```python
from build123d import *

# Parameters (mm, degrees)
BOSS_EXTRUDE1_DEPTH = 50
CUT_EXTRUDE1_REACH  = 9
SKETCH3_R           = 2.5


with BuildPart() as part:
    # Sketch2 → Boss-Extrude1 (new body)
    with BuildSketch(Plane.XY):
        Polygon((-15.713485752, 63.637116303), (-18.483485752, 60.867117128), (-15.713485752, 58.097116303), (-15.713485752, 51.097116303), (-22.713485752, 51.097116303), (-22.713485752, 65.637116303), (-15.713485752, 65.637116303), align=None)
    extrude(amount=BOSS_EXTRUDE1_DEPTH)

    # Sketch3 → Cut-Extrude1 (cut, up to next)
    with BuildSketch(Plane.ZY.offset(22.713485752), mode=Mode.PRIVATE) as cut_extrude1_sk1:
        with Locations((17, 55.097116303)):
            Circle(SKETCH3_R)
    cut_extrude1_tool1 = extrude(cut_extrude1_sk1.sketch, amount=-CUT_EXTRUDE1_REACH, mode=Mode.PRIVATE) & part.part
    add(cut_extrude1_tool1.solids().sort_by_distance((-22.713486, 55.097116, 17))[0], mode=Mode.SUBTRACT)
    # Sketch3 → Cut-Extrude1 (cut, up to next)
    with BuildSketch(Plane.ZY.offset(22.713485752), mode=Mode.PRIVATE) as cut_extrude1_sk2:
        with Locations((33, 55.097116303)):
            Circle(SKETCH3_R)
    cut_extrude1_tool2 = extrude(cut_extrude1_sk2.sketch, amount=-CUT_EXTRUDE1_REACH, mode=Mode.PRIVATE) & part.part
    add(cut_extrude1_tool2.solids().sort_by_distance((-22.713486, 55.097116, 33))[0], mode=Mode.SUBTRACT)


solid = part.part
```
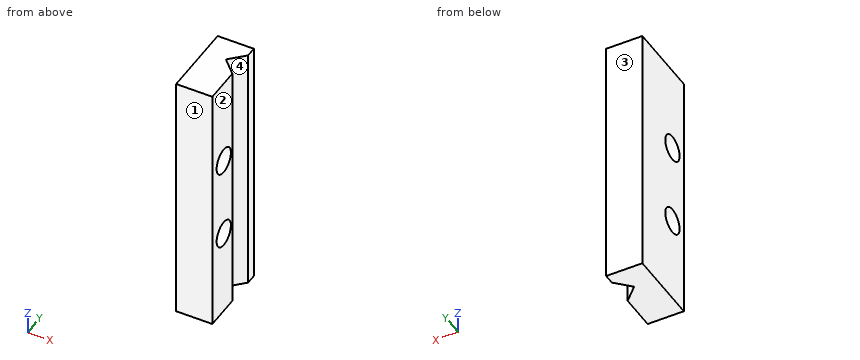
Read the model definition and answer for the solid it produces. Units are mm, in the model's axes. Face numbers are marked on the shaded views. Coordinates: 2 decimals unless noted, no trailing zeros. Loops run counter-clockwise (first coordinate to the right, second up) from the corner with the lowest first, then second, coordinate; pieces in that order, holes last.
(1) Consider line 1 along Y through (x, z) = (-20.5, 17); line 2 along Z through (x, y) = (-18.75, 53.25); line 3 along Z through (x, y) = (-17.25, 54.25). Determine where each line is inside the solid, lowest interval first.
Solution:
line 1: y = 51.1 to 52.6, 57.6 to 65.64
line 2: z = 0 to 15.32, 18.68 to 31.32, 34.68 to 50
line 3: z = 0 to 14.65, 19.35 to 30.65, 35.35 to 50
(2) The mould has two halves that part along Y. Classify the marked faces 1, 2, 3 and 4: released by +Y, released by -Y, zero draft, split by the parting line, or undercut.
Solution:
face 1: released by -Y
face 2: zero draft
face 3: released by +Y
face 4: undercut
(3) The part is cut by section C-C (z = 12). Determine the outline of the cut face in (x, y), and give its area (3 significant figures).
Solution:
outline: (-22.71, 51.1) - (-15.71, 51.1) - (-15.71, 58.1) - (-18.48, 60.87) - (-15.71, 63.64) - (-15.71, 65.64) - (-22.71, 65.64) - close
area: 94.1 mm2
(4) The part is cut by section D-D (y = 62.25). Determine the outline of the cut face in (x, z).
Solution:
outline: (-22.71, 0) - (-17.1, 0) - (-17.1, 50) - (-22.71, 50) - close
(5) The part is cut by section B-B (x = -19.75). Determine the outline of the cut face in (y, z).
Solution:
outline: (51.1, 0) - (65.64, 0) - (65.64, 50) - (51.1, 50) - close; hole circle Ø5 at (55.1, 17); hole circle Ø5 at (55.1, 33)
(6) The part is cut by section A-A (z = 33). Determine the outline of the cut face in (x, y).
Solution:
outline: (-22.71, 51.1) - (-15.71, 51.1) - (-15.71, 52.6) - (-22.71, 52.6) - close; (-22.71, 57.6) - (-15.71, 57.6) - (-15.71, 58.1) - (-18.48, 60.87) - (-15.71, 63.64) - (-15.71, 65.64) - (-22.71, 65.64) - close
